from build123d import *

# Parameters (mm, degrees)
SKETCH1_R           = 69.85
BOSS_EXTRUDE1_DEPTH = 3.81
SKETCH2_R           = 69.85
SKETCH2_R_2         = 63.881
SKETCH2_R_3         = 56.6547
SKETCH2_R_4         = 51.181
BOSS_EXTRUDE2_DEPTH = 10.16
SKETCH3_R           = 12.827
SKETCH3_R_2         = 10.3378
BOSS_EXTRUDE3_DEPTH = 3.81
CUT_EXTRUDE1_DEPTH  = 3.81
SKETCH5_R           = 12.7
CUT_EXTRUDE2_DEPTH  = 10.16
SKETCH6_W           = 139.7
SKETCH6_H           = 139.7
BOSS_EXTRUDE4_DEPTH = 3.048
SKETCH7_R           = 7.62
SKETCH7_R_2         = 2.54
CUT_EXTRUDE3_DEPTH  = 3.048


with BuildPart() as part:
    # Sketch1 → Boss-Extrude1 (new body)
    with BuildSketch(Plane(origin=(0, 0, 0), x_dir=(1, 0, 0), z_dir=(0, 1, 0))):
        Circle(SKETCH1_R)
    extrude(amount=BOSS_EXTRUDE1_DEPTH)

    # Sketch2 → Boss-Extrude2 (add)
    with BuildSketch(Plane(origin=(0, 3.81, 0), x_dir=(1, 0, 0), z_dir=(0, 1, 0))):
        Circle(SKETCH2_R)
        Circle(SKETCH2_R_2, mode=Mode.SUBTRACT)
        Circle(SKETCH2_R_3)
        Circle(SKETCH2_R_4, mode=Mode.SUBTRACT)
    extrude(amount=BOSS_EXTRUDE2_DEPTH)

    # Sketch3 → Boss-Extrude3 (add)
    with BuildSketch(Plane(origin=(0, 3.81, 0), x_dir=(1, 0, 0), z_dir=(0, 1, 0))):
        Circle(SKETCH3_R)
        Circle(SKETCH3_R_2, mode=Mode.SUBTRACT)
    extrude(amount=BOSS_EXTRUDE3_DEPTH)

    # Sketch4 → Cut-Extrude1 (cut)
    with BuildSketch(Plane(origin=(0, 7.62, 0), x_dir=(1, 0, 0), z_dir=(0, 1, 0))):
        with BuildLine():
            Line((4.238603881, -9.428910116), (5.259201376, -11.699261938))
            ThreePointArc((5.259201376, -11.699261938), (8.835496643, -9.29870572), (11.415504655, -5.849630969))
            Line((11.415504655, -5.849630969), (9.200218603, -4.714455058))
            ThreePointArc((9.200218603, -4.714455058), (7.120885413, -7.494204412), (4.238603881, -9.428910116))
        make_face()
    extrude(amount=-CUT_EXTRUDE1_DEPTH, mode=Mode.SUBTRACT)

    # Sketch5 → Cut-Extrude2 (cut)
    with BuildSketch(Plane(origin=(0, 3.81, 0), x_dir=(1, 0, 0), z_dir=(0, 1, 0))):
        with Locations((25.4, -24.886815787)):
            Circle(SKETCH5_R)
    extrude(amount=-CUT_EXTRUDE2_DEPTH, mode=Mode.SUBTRACT)

    # Sketch6 → Boss-Extrude4 (add)
    with BuildSketch(Plane.XZ):
        Rectangle(SKETCH6_W, SKETCH6_H)
    extrude(amount=BOSS_EXTRUDE4_DEPTH)

    # Sketch7 → Cut-Extrude3 (cut)
    with BuildSketch(Plane(origin=(0, 0, 0), x_dir=(1, 0, 0), z_dir=(0, 1, 0))):
        with Locations((25.4, -24.886815787)):
            Circle(SKETCH7_R)
        with Locations((-66.04, -66.04)):
            Circle(SKETCH7_R_2)
        with Locations((66.04, -66.04)):
            Circle(SKETCH7_R_2)
        with Locations((66.04, 66.04)):
            Circle(SKETCH7_R_2)
        with Locations((-66.04, 66.04)):
            Circle(SKETCH7_R_2)
    extrude(amount=-CUT_EXTRUDE3_DEPTH, mode=Mode.SUBTRACT)


solid = part.part
For this review, take the finished solid that the model builds, in its own axes (mm). A direction names the side the tool comes from. Give positions to 0.01 mm unless a question says otherwise; leave off trailing zeros. Loops run counter-clockwise (first coordinate to the right, second up) from the corner with the lowest first, then second, coordinate; pieces in that order, holes last. Notation, with made-up numbers: M 52.5,31.25 L 98.5,31.25 A24 cw 98.5,66.25 Z; hole C 6,-33.5 d11. An arc over 180 degrees is marked long. Answer as a JSON object with one key per item and string values. Group by question number.
Q1. Add section A-A on z = 20. Give the boundary of the cut face in (x, y), and give its area (3 significant figures).
Q2. For probe 1 along X at (y, z) = (6.15, 0); probe 2 along Z at (x, y) = (66.04, -2.05); probe 3 along X at (y, z) = (8.75, 0), list the stretches that pass through material, from the lowest coordinate up. Write a range as [from, to].
Q3. Add section C-C on z = 66.04. Give the boundary of the cut face in (x, y), and give its area (3 significant figures).
Q4. Add section B-B on x = -66.04. Give the boundary of the cut face in (y, z), and give its area (3 significant figures).
Q5. Insertion check: P1, Ø1, axis at x = -45.5, y = 2, coming from the +Z side; P2, Ø5, axis at y = 5, z = -13, coming from the +X side; P3, Ø6, axis at x = 35.5, y = 6, coming from the -Z side. Each pin has a flat end and moves straight along its axis. Give the tip position at first contact, or say it passes through.
Q6. Tool access review of faces 1 (the flat face through (-38.2, 3.81, 42.3)), 2 (the flat face through (31, 13.97, 57)), 3 (the flat face through (-53, 0, 53)): name each direction out of +Z, -Z, +X, -X, +Y, -Y from which nothing blocks a thin tool from reaching the whole face with its end or side.
Q7. Mouldability with a two-part tool opening along X and no side actions: class faces 4 (the cylindrical face through (-55.431, 6.887, 42.503)), 5 (the cylindrical face through (-63.694, -1.503, 67.013)), 6 (the flat face through (53, 0, 53)) as +X half, -X half, draft (parallel to the pull), parting line (faces both ways), or undercut.
Q8. Add section D-D on x = -14.5. Give the boundary of the cut face in (y, z), and give its area (3 significant figures).
Checked values:
{
 "1": {"outline": "M -69.85,-3.05 L 19.55,-3.05 L 19.55,0 L 13.68,0 L 13.68,3.81 L -47.11,3.81 L -47.11,13.97 L -53.01,13.97 L -53.01,3.81 L -60.67,3.81 L -60.67,13.97 L -66.93,13.97 L -66.93,0 L -69.85,0 Z; M 31.25,-3.05 L 69.85,-3.05 L 69.85,0 L 66.93,0 L 66.93,13.97 L 60.67,13.97 L 60.67,3.81 L 53.01,3.81 L 53.01,13.97 L 47.11,13.97 L 47.11,3.81 L 37.12,3.81 L 37.12,0 L 31.25,0 Z", "area": "1,060 mm²"},
 "2": {"probe 1": "[-69.85, -63.88], [-56.65, -51.18], [-12.83, -10.34], [10.34, 12.83], [51.18, 56.65], [63.88, 69.85]", "probe 2": "[-69.85, -68.58], [-63.5, 63.5], [68.58, 69.85]", "probe 3": "[-69.85, -63.88], [-56.65, -51.18], [51.18, 56.65], [63.88, 69.85]"},
 "3": {"outline": "M -69.85,-3.05 L -68.58,-3.05 L -68.58,0 L -69.85,0 Z; M -63.5,-3.05 L 63.5,-3.05 L 63.5,0 L 22.75,0 L 22.75,13.97 L -22.75,13.97 L -22.75,0 L -63.5,0 Z; M 68.58,-3.05 L 69.85,-3.05 L 69.85,0 L 68.58,0 Z", "area": "1,030 mm²"},
 "4": {"outline": "M -3.05,-69.85 L 0,-69.85 L 0,-68.58 L -3.05,-68.58 Z; M -3.05,-63.5 L 0,-63.5 L 0,-22.75 L 13.97,-22.75 L 13.97,22.75 L 0,22.75 L 0,63.5 L -3.05,63.5 Z; M -3.05,68.58 L 0,68.58 L 0,69.85 L -3.05,69.85 Z", "area": "1,030 mm²"},
 "5": {"P1": "z = 53.42", "P2": "x = 69.06", "P3": "z = -61.83"},
 "6": {"face 1": "+Y", "face 2": "+Z, -Z, +X, -X, +Y", "face 3": "+Z, -X, +Y"},
 "7": {"face 4": "parting line", "face 5": "undercut", "face 6": "draft"},
 "8": {"outline": "M -3.05,-69.85 L 0,-69.85 L 0,-68.33 L 13.97,-68.33 L 13.97,-62.21 L 3.81,-62.21 L 3.81,-54.77 L 13.97,-54.77 L 13.97,-49.08 L 3.81,-49.08 L 3.81,49.08 L 13.97,49.08 L 13.97,54.77 L 3.81,54.77 L 3.81,62.21 L 13.97,62.21 L 13.97,68.33 L 0,68.33 L 0,69.85 L -3.05,69.85 Z", "area": "1,190 mm²"}
}
